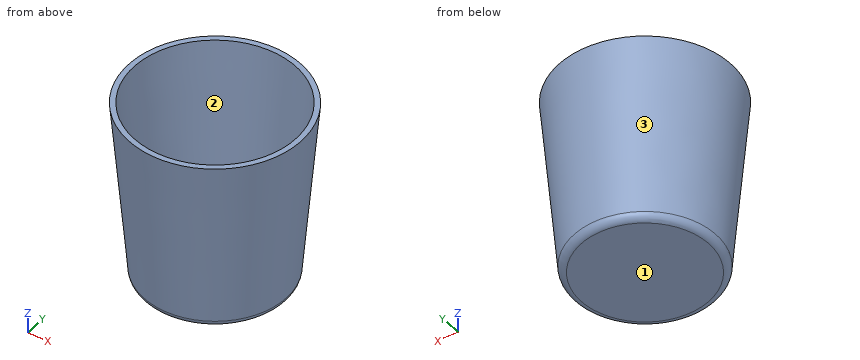
from build123d import *

# Parameters (mm, degrees)
F1_T = -1.5
F2_R = 5
F4_R = 2


with BuildPart() as f3:
    # F0 (on Front) → F3 (revolve)
    with BuildSketch(Plane.XZ):
        Polygon((-20, 0), (0, 0), (0, 50.6066906631), (-24.4275117316, 50.6066906631), align=None)
    revolve(axis=Axis((0, 0, 25.3033453315), (0, 0, -1)))

    # F1
    f1_openings = [f3.faces().sort_by_distance(p)[0] for p in [
        (0, 0, 50.606691),
    ]]
    offset(amount=F1_T, openings=f1_openings)

    # F2
    f2_edges = [f3.edges().sort_by_distance(p)[0] for p in [
        (18.625503, 0, 1.5),
    ]]
    fillet(f2_edges, radius=F2_R)

    # F4
    f4_edges = [f3.edges().sort_by_distance(p)[0] for p in [
        (20, 0, 0),
    ]]
    fillet(f4_edges, radius=F4_R)


solid = f3.part
Geometry: final body of the model. Coordinates: model frame, mm. Face numbers are marked on the shaded views. Round coordinates to 2 decimals unless told otherwise and drop trailing zeros. Order: outer loops, then holes, each group sorted by start corner. A loop starts at its lowest first (then second) coordinate and runs counter-clockwise, first axis right, second up. Notation, with made-up numbers: (-32.5, 25) - (0.5, 25) arc R34 ccw to (0.5, 55) - close; hole circle Ø1 at (24, -7.5). An arc over 180 degrees is marked (long way). Write each question's results on one line, items separated by ' | '.
Item 1: Section A-A, the plane y = 0. Return the cut outline in (x, z).
Completed:
outline: (-24.43, 50.61) - (-20.16, 1.83) arc R2 ccw to (-18.17, 0) - (18.17, 0) arc R2 ccw to (20.16, 1.83) - (24.43, 50.61) - (22.92, 50.61) - (19.02, 6.06) arc R5 cw to (14.04, 1.5) - (-14.04, 1.5) arc R5 cw to (-19.02, 6.06) - (-22.92, 50.61) - close
Item 2: Section D-D, the plane z = 24.5. Return the cut outline in (x, y), and give its area (3 significant figures).
Completed:
outline: circle Ø44.29 at (0, 0); hole circle Ø41.28 at (0, 0) | area: 202 mm^2
Item 3: First-contact query: pin 1 Ø6 at (y, z) = (-11, 35) entering from +X; pin 2 Ø1.5 at (x, z) = (5.5, 15) entering from +Y; pin 3 Ø6 at (x, z) = (-1, 41.5) entering from +Y. Flat tips, straight axial feed; report the tip coordinate or a pass-through.
Completed:
pin 1: x = 21.66 | pin 2: y = 20.79 | pin 3: y = 23.88
Item 4: Mould query, pull axis X, two halves, no side actions, for the marked faces 1, 2 and 3. Classes: pulls with the +X half, pulls with the -X half, needs draft (parallel to the pull), parting line crosses it, or undercut.
Completed:
face 1: needs draft | face 2: undercut | face 3: parting line crosses it
Item 5: Material intervals for line 1 along Y through (x, z) = (16, 24); line 2 along Y through (x, z) = (8.5, 21.5); line 3 along X through (y, z) = (-4, 27), sorted ascending. Write a range as [from, to].
Completed:
line 1: [-15.24, -12.97], [12.97, 15.24] | line 2: [-20.16, -18.52], [18.52, 20.16] | line 3: [-22, -20.47], [20.47, 22]
Item 6: Section C-C, the plane z = 17. Return the cut outline in (x, y).
Completed:
outline: circle Ø42.97 at (0, 0); hole circle Ø39.96 at (0, 0)
